```python
from build123d import *

# Parameters (mm, degrees)
SKETCH1_W           = 20.78
SKETCH1_H           = 27.15
SKETCH1_R           = 0.33
SKETCH1_W_2         = 7.49
SKETCH1_H_2         = 16.35
BOSS_EXTRUDE1_DEPTH = 0.85


with BuildPart() as part:
    # Sketch1 → Boss-Extrude1 (new body)
    with BuildSketch(Plane(origin=(0, 0, 0), x_dir=(1, 0, 0), z_dir=(0, 1, 0))):
        with Locations((10.39, 13.575)):
            Rectangle(SKETCH1_W, SKETCH1_H)
        with Locations(Location((2.389, 23.96, 0), (0, 0, 270))):
            Circle(SKETCH1_R, mode=Mode.SUBTRACT)
        with Locations(Location((4.169, 23.96, 0), (0, 0, 270))):
            Circle(SKETCH1_R, mode=Mode.SUBTRACT)
        with Locations(Location((5.949, 23.96, 0), (0, 0, 270))):
            Circle(SKETCH1_R, mode=Mode.SUBTRACT)
        with Locations(Location((7.729, 23.96, 0), (0, 0, 270))):
            Circle(SKETCH1_R, mode=Mode.SUBTRACT)
        with Locations(Location((9.509, 23.96, 0), (0, 0, 270))):
            Circle(SKETCH1_R, mode=Mode.SUBTRACT)
        with Locations(Location((11.289, 23.96, 0), (0, 0, 270))):
            Circle(SKETCH1_R, mode=Mode.SUBTRACT)
        with Locations(Location((13.069, 23.96, 0), (0, 0, 270))):
            Circle(SKETCH1_R, mode=Mode.SUBTRACT)
        with Locations(Location((14.849, 23.96, 0), (0, 0, 270))):
            Circle(SKETCH1_R, mode=Mode.SUBTRACT)
        with Locations(Location((16.629, 23.96, 0), (0, 0, 270))):
            Circle(SKETCH1_R, mode=Mode.SUBTRACT)
        with Locations(Location((18.409, 23.96, 0), (0, 0, 270))):
            Circle(SKETCH1_R, mode=Mode.SUBTRACT)
        with Locations(Location((18.409, 3.19, 0), (0, 0, 90))):
            Circle(SKETCH1_R, mode=Mode.SUBTRACT)
        with Locations(Location((16.629, 3.19, 0), (0, 0, 90))):
            Circle(SKETCH1_R, mode=Mode.SUBTRACT)
        with Locations(Location((14.849, 3.19, 0), (0, 0, 90))):
            Circle(SKETCH1_R, mode=Mode.SUBTRACT)
        with Locations(Location((13.069, 3.19, 0), (0, 0, 90))):
            Circle(SKETCH1_R, mode=Mode.SUBTRACT)
        with Locations(Location((11.289, 3.19, 0), (0, 0, 90))):
            Circle(SKETCH1_R, mode=Mode.SUBTRACT)
        with Locations(Location((9.509, 3.19, 0), (0, 0, 90))):
            Circle(SKETCH1_R, mode=Mode.SUBTRACT)
        with Locations(Location((7.729, 3.19, 0), (0, 0, 90))):
            Circle(SKETCH1_R, mode=Mode.SUBTRACT)
        with Locations(Location((5.949, 3.19, 0), (0, 0, 90))):
            Circle(SKETCH1_R, mode=Mode.SUBTRACT)
        with Locations(Location((4.169, 3.19, 0), (0, 0, 90))):
            Circle(SKETCH1_R, mode=Mode.SUBTRACT)
        with Locations(Location((2.389, 3.19, 0), (0, 0, 90))):
            Circle(SKETCH1_R, mode=Mode.SUBTRACT)
        with Locations((15.135, 13.575)):
            Rectangle(SKETCH1_W_2, SKETCH1_H_2, mode=Mode.SUBTRACT)
        with Locations((5.645, 13.575)):
            Rectangle(SKETCH1_W_2, SKETCH1_H_2, mode=Mode.SUBTRACT)
    extrude(amount=BOSS_EXTRUDE1_DEPTH)


solid = part.part
```
Could you check a few things on this model? Use its own coordinates, in mm. A direction names the side the tool comes from. Round coordinates to 2 decimals unless told otherwise and drop trailing zeros. Loops run counter-clockwise (first coordinate to the right, second up) from the corner with the lowest first, then second, coordinate; pieces in that order, holes last. Notation, with made-up numbers: (73, 75.5) - (101, 75.5) arc R20 ccw to (101, 100.5) - close; hole circle Ø10 at (21.25, 72.25). An arc over 180 degrees is marked (long way). Answer as CSV lines item,"result".
1. Please list where these lines run through material, in increasing order: line 1 along X through (y, z) = (0.7, -12.5); line 2 along Z through (x, y) = (11.25, 0.4); line 3 along Z through (x, y) = (9.25, 0.45). Write a range as [from, to].
Filled in:
line 1,"x = [0, 1.9], [9.39, 11.39], [18.88, 20.78]"
line 2,"z = [-27.15, -24.29], [-23.63, -3.52], [-2.86, 0]"
line 3,"z = [-27.15, -24.16], [-23.76, -21.75], [-5.4, -3.39], [-2.99, 0]"
2. I want a section at B-B on x = 3.5. List the corners of the cut face in (y, z) for me.
Filled in:
outline,"(0, -27.15) - (0.85, -27.15) - (0.85, -21.75) - (0, -21.75) - close; (0, -5.4) - (0.85, -5.4) - (0.85, 0) - (0, 0) - close"
3. I want a section at C-C on z = -23.96. Count the separate pieces of the cut face and the enclosed holes in it, then the cut area to 3 significant figures.
Filled in:
separate pieces,"11"
enclosed holes,"0"
area,"12.1 mm^2"
4. On a 3-axis mill with a long thin cutter (end or side, diameter ignored), from which of +Z, -Z, +X, -X, +Y, -Y can I reach the whole of each face in a straight line? I mean faces 4 (the face through (20.78, 0.4, -13.4)), 5 (the face through (5.6, 0.4, -21.75)). Say none if no direction works.
Filled in:
face 4,"+Z, -Z, +X, +Y, -Y"
face 5,"+Y, -Y"
5. I want a section at A-A on z = -11. List the corners of the cut face in (x, y) for me, then the cut area to 3 significant figures.
Filled in:
outline,"(0, 0) - (1.9, 0) - (1.9, 0.85) - (0, 0.85) - close; (9.39, 0) - (11.39, 0) - (11.39, 0.85) - (9.39, 0.85) - close; (18.88, 0) - (20.78, 0) - (20.78, 0.85) - (18.88, 0.85) - close"
area,"4.93 mm^2"
6. We'd pull the mould along Z, two halves only. Please class faces 1 (the face through (10.2, 0.4, 0)), 2 (the face through (1.9, 0.4, -13.5)), 3 (the face through (10, 0.85, -14)): +Z half, -Z half, draft (parallel to the pull), parting line (faces both ways), or undercut.
Filled in:
face 1,"+Z half"
face 2,"undercut"
face 3,"draft"
